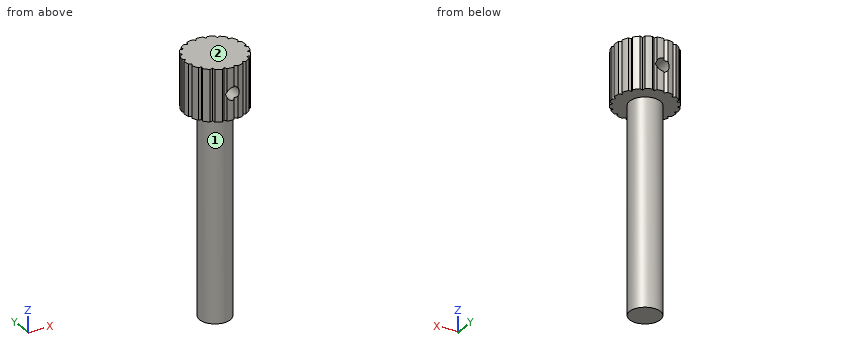
```python
from build123d import *

# Parameters (mm, degrees)
F1_DEPTH = 20
F3_R     = 2.5
F4_DEPTH = 48.262108
F5_R     = 6
F6_DEPTH = 80


with BuildPart() as f1:
    # F0 (on Top) → F1 (new body)
    with BuildSketch(Plane.XY):
        with BuildLine():
            Line((-10.553502, 21.159582), (-11.701467, 21.747872))
            ThreePointArc((-11.701467, 21.747872), (-12.807584, 21.051104), (-13.831344, 20.23815))
            Line((-13.831344, 20.23815), (-13.656418, 18.96014))
            Line((-13.656418, 18.96014), (-14.936359, 19.120325))
            ThreePointArc((-14.936359, 19.120325), (-15.73746, 18.087264), (-16.421432, 16.97319))
            Line((-16.421432, 16.97319), (-15.819951, 15.832082))
            Line((-15.819951, 15.832082), (-17.077488, 15.544841))
            ThreePointArc((-17.077488, 15.544841), (-17.476949, 14.300088), (-17.738638, 13.019269))
            Line((-17.738638, 13.019269), (-16.783148, 12.152696))
            Line((-16.783148, 12.152696), (-17.866604, 11.452675))
            ThreePointArc((-17.866604, 11.452675), (-17.816244, 10.146366), (-17.624085, 8.853287))
            Line((-17.624085, 8.853287), (-16.429833, 8.365772))
            Line((-16.429833, 8.365772), (-17.208528, 7.337403))
            ThreePointArc((-17.208528, 7.337403), (-16.714421, 6.127099), (-16.091591, 4.977724))
            Line((-16.091591, 4.977724), (-14.802622, 4.928068))
            Line((-14.802622, 4.928068), (-15.182632, 3.695388))
            ThreePointArc((-15.182632, 3.695388), (-14.304375, 2.727069), (-13.325997, 1.86003))
            Line((-13.325997, 1.86003), (-12.097779, 2.254223))
            Line((-12.097779, 2.254223), (-12.033271, 0.965911))
            ThreePointArc((-12.033271, 0.965911), (-10.876794, 0.35637), (-9.660875, -0.123755))
            Line((-9.660875, -0.123755), (-8.641549, 0.66674))
            Line((-8.641549, 0.66674), (-8.140303, -0.521814))
            ThreePointArc((-8.140303, -0.521814), (-6.845095, -0.699057), (-5.538292, -0.734358))
            Line((-5.538292, -0.734358), (-4.850804, 0.357095))
            Line((-4.850804, 0.357095), (-3.973277, -0.588344))
            ThreePointArc((-3.973277, -0.588344), (-2.695559, -0.311911), (-1.455493, 0.101869))
            Line((-1.455493, 0.101869), (-1.182765, 1.362634))
            Line((-1.182765, 1.362634), (-0.0348, 0.774344))
            ThreePointArc((-0.0348, 0.774344), (1.071317, 1.471112), (2.095076, 2.284066))
            Line((2.095076, 2.284066), (1.92015, 3.562076))
            Line((1.92015, 3.562076), (3.200092, 3.401891))
            ThreePointArc((3.200092, 3.401891), (4.001193, 4.434952), (4.685165, 5.549026))
            Line((4.685165, 5.549026), (4.083684, 6.690134))
            Line((4.083684, 6.690134), (5.341221, 6.977375))
            ThreePointArc((5.341221, 6.977375), (5.740682, 8.222128), (6.002371, 9.502947))
            Line((6.002371, 9.502947), (5.046881, 10.36952))
            Line((5.046881, 10.36952), (6.130337, 11.069541))
            ThreePointArc((6.130337, 11.069541), (6.079977, 12.37585), (5.887818, 13.668929))
            Line((5.887818, 13.668929), (4.693566, 14.156444))
            Line((4.693566, 14.156444), (5.472261, 15.184813))
            ThreePointArc((5.472261, 15.184813), (4.978154, 16.395117), (4.355324, 17.544492))
            Line((4.355324, 17.544492), (3.066354, 17.594148))
            Line((3.066354, 17.594148), (3.446365, 18.826828))
            ThreePointArc((3.446365, 18.826828), (2.568108, 19.795147), (1.58973, 20.662186))
            Line((1.58973, 20.662186), (0.361512, 20.267993))
            Line((0.361512, 20.267993), (0.297004, 21.556305))
            ThreePointArc((0.297004, 21.556305), (-0.859473, 22.165846), (-2.075392, 22.645971))
            Line((-2.075392, 22.645971), (-3.094718, 21.855476))
            Line((-3.094718, 21.855476), (-3.595965, 23.04403))
            ThreePointArc((-3.595965, 23.04403), (-4.891172, 23.221273), (-6.197975, 23.256574))
            Line((-6.197975, 23.256574), (-6.885463, 22.165121))
            Line((-6.885463, 22.165121), (-7.76299, 23.11056))
            ThreePointArc((-7.76299, 23.11056), (-9.040708, 22.834127), (-10.280774, 22.420347))
            Line((-10.280774, 22.420347), (-10.553502, 21.159582))
        make_face()
    extrude(amount=F1_DEPTH)

    # F3 (on offset) → F4 (cut, through all)
    with BuildSketch(Plane.XZ.offset(25)):
        with Locations((-5.868134, 10)):
            Circle(F3_R)
    extrude(amount=-F4_DEPTH, mode=Mode.SUBTRACT)

    # F5 (on face) → F6 (join)
    with BuildSketch(Plane(origin=(0, 0, 0), x_dir=(1, 0, 0), z_dir=(0, 0, -1))):
        with Locations((-5.868134, -11.261108)):
            Circle(F5_R)
    extrude(amount=F6_DEPTH)


solid = f1.part
```
For this review, take the finished solid that the model builds, in its own axes (mm). Face numbers are marked on the shaded views. A direction names the side the tool comes from. Coordinates: 2 decimals unless noted, no trailing zeros. Order: outer loops, then holes, each group sorted by start corner. A loop starts at its lowest first (then second) coordinate and runs counter-clockwise, first axis right, second up. Notation, with made-up numbers: (14.25, 66) - (21.25, 66) arc R14 ccw to (21.25, 83) - close; hole circle Ø8 at (-23, -17.5). An arc over 180 degrees is marked (long way). Answer as a JSON object with one key per item and string values. Group by question number.
1. We need section A-A on z = -42.5. State the section outline as (x, y) points.
2. For probe 1 along X at (y, z) = (13, 10); probe 2 along Z at (x, y) = (-6, 15.5); probe 3 along Z at (x, y) = (1.5, 7.5), list the stretches that pass through material, from the lowest coordinate up.
3. For the marked faces 1 and 2, list the 3-axis set-ups (+Z, -Z, +X, -X, +Y, -Y) from which the entire face can be reached by the end or side of a thin tool; tool diameter is ignored.
4. Clearance check with flat-ended pins moving along their axes: P1, Ø3, axis at y = 7, z = -58.5, coming from the +X side; P2, Ø2, axis at x = -6, z = -13, coming from the +Y side; P3, Ø6, axis at x = -5.87, z = 10, coming from the +Y side; P4, Ø12, axis at y = 15.5, z = -36, coming from the -X side. State where each tip first meets the part, or that it passes through.
Final values:
{
 "1": {"outline": "circle Ø12 at (-5.87, 11.26)"},
 "2": {"probe 1": "-17.72 to -8.37, -3.37 to 6.01", "probe 2": "-80 to 7.5, 12.5 to 20", "probe 3": "0 to 20"},
 "3": {"face 1": "-Z", "face 2": "+Z, +X, -X, +Y, -Y"},
 "4": {"P1": "x = -0.54", "P2": "y = 17.26", "P3": "y = 23.26", "P4": "x = -11.87"}
}
